Verification items for the finished model (mm, model axes). Give positions to 0.01 mm unless a question says otherwise; leave off trailing zeros. Write each loop counter-clockwise with the first axis right and the second up, starting at its lowest first coordinate (ties: lowest second). Pieces come first, ordered by that corner, then holes. Notation, with made-up numbers: (85.25, 78) - (119.25, 78) arc R36 ccw to (119.25, 116) - close; hole circle Ø10 at (-27, 52.25). An arc over 180 degrees is marked (long way). Put each result on its own line as item: value.
from build123d import *

# Parameters (mm, degrees)
F0_R     = 1
F0_R_2   = 0.8
F1_DEPTH = 1
F2_R     = 1


with BuildPart() as f1:
    # F0 (on Top) → F1 (new body)
    with BuildSketch(Plane.XY):
        Polygon((14.0690184001, 25), (0, 25), (-14.0690184001, 25), (-26.7296075576, 13.6899425008), (-24.0647631939, 10.7068896154), (-12.5425545984, 21), (0, 21), (12.5425545984, 21), (24.0647631939, 10.7068896154), (26.7296075576, 13.6899425008), align=None)
        with Locations((0, 23)):
            Circle(F0_R, mode=Mode.SUBTRACT)
        Polygon((28.9542586869, 11.7025995837), (26.7296075576, 13.6899425008), (24.0647631939, 10.7068896154), (26.2894143232, 8.7195466983), align=None)
        Polygon((-24.0647631939, 10.7068896154), (-26.7296075576, 13.6899425008), (-28.9542586869, 11.7025995837), (-26.2894143232, 8.7195466983), align=None)
        Polygon((31.3294992745, 9.5807309025), (28.9542586869, 11.7025995837), (26.2894143232, 8.7195466983), (27.3294992745, 7.7904097951), (27.3294992745, 0.0814010352), (27.3294992745, -0.0814010352), (27.3294992745, -7.7904097951), (26.2894143232, -8.7195466983), (28.9542586869, -11.7025995837), (31.3294992745, -9.5807309025), (31.3294992745, 0), align=None)
        with Locations((29.25, -7.3612159322)):
            Circle(F0_R_2, mode=Mode.SUBTRACT)
        with Locations((29.25, 7.3612159322)):
            Circle(F0_R_2, mode=Mode.SUBTRACT)
        Polygon((26.2894143232, 8.7195466983), (24.0647631939, 10.7068896154), (14.5, 0), (24.0647631939, -10.7068896154), (26.2894143232, -8.7195466983), (18.5, 0), align=None)
        with Locations((16.5, 0)):
            Circle(F0_R_2, mode=Mode.SUBTRACT)
        Polygon((-26.2894143232, 8.7195466983), (-28.9542586869, 11.7025995837), (-31.3294992745, 9.5807309025), (-31.3294992745, 0), (-31.3294992745, -9.5807309025), (-28.9542586869, -11.7025995837), (-26.2894143232, -8.7195466983), (-27.3294992745, -7.7904097951), (-27.3294992745, -0.0814010352), (-27.3294992745, 0.0814010352), (-27.3294992745, 7.7904097951), align=None)
        with Locations((-29.25, -7.3612159322)):
            Circle(F0_R_2, mode=Mode.SUBTRACT)
        with Locations((-29.25, 7.3612159322)):
            Circle(F0_R_2, mode=Mode.SUBTRACT)
        Polygon((-14.5, 0), (-24.0647631939, 10.7068896154), (-26.2894143232, 8.7195466983), (-18.5, 0), (-26.2894143232, -8.7195466983), (-24.0647631939, -10.7068896154), align=None)
        with Locations((-16.5, 0)):
            Circle(F0_R_2, mode=Mode.SUBTRACT)
        Polygon((26.2894143232, -8.7195466983), (24.0647631939, -10.7068896154), (26.7296075576, -13.6899425008), (28.9542586869, -11.7025995837), align=None)
        Polygon((26.7296075576, -13.6899425008), (24.0647631939, -10.7068896154), (12.5425545984, -21), (0, -21), (-12.5425545984, -21), (-24.0647631939, -10.7068896154), (-26.7296075576, -13.6899425008), (-14.0690184001, -25), (0, -25), (14.0690184001, -25), align=None)
        with Locations((0, -23)):
            Circle(F0_R, mode=Mode.SUBTRACT)
        Polygon((-26.7296075576, -13.6899425008), (-24.0647631939, -10.7068896154), (-26.2894143232, -8.7195466983), (-28.9542586869, -11.7025995837), align=None)
    extrude(amount=F1_DEPTH)

    # F2
    f2_edges = [f1.edges().sort_by_distance(p)[0] for p in [
        (-14.069018, 25, 0.5),
        (-31.329499, 9.580731, 0.5),
        (-31.329499, -9.580731, 0.5),
        (-14.069018, -25, 0.5),
        (14.069018, -25, 0.5),
        (31.329499, -9.580731, 0.5),
        (31.329499, 9.580731, 0.5),
        (14.069018, 25, 0.5),
        (14.5, 0, 0.5),
        (-14.5, 0, 0.5),
    ]]
    fillet(f2_edges, radius=F2_R)


solid = f1.part
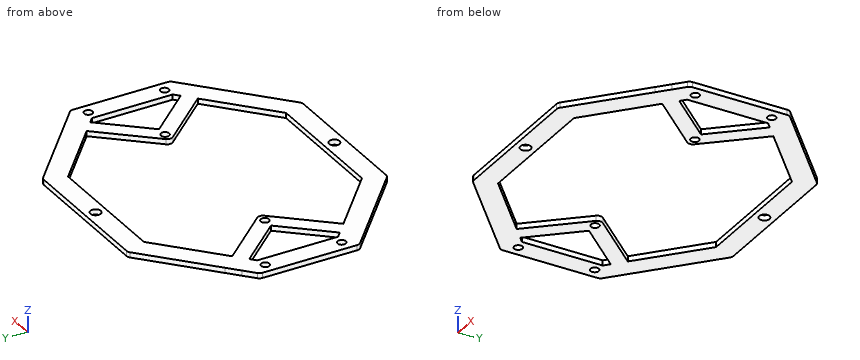
Q1. Section check D-D, the plane y = -4. Record the cut outline in (x, z), plus the area to 3 significant figures.
Answers follow:
outline: (-31.33, 0) - (-27.33, 0) - (-27.33, 1) - (-31.33, 1) - close; (-22.07, 0) - (-18.07, 0) - (-18.07, 1) - (-22.07, 1) - close; (18.07, 0) - (22.07, 0) - (22.07, 1) - (18.07, 1) - close; (27.33, 0) - (31.33, 0) - (31.33, 1) - (27.33, 1) - close
area: 16.0 mm2
Q2. Go/stop test with a flat-tipped pin: pin 1 Ø1 at (x, y) = (16.5, 0) entering from +Z. Record where the tip stops, or that it passes through.
Answers follow:
pin 1: passes through
Q3. Scan lines: line 1 along Y through (x, z) = (0, 0.25); line 2 along X through (y, z) = (-4, 0.55); line 3 along Y through (x, z) = (-8, 0.25). Record each from-to range of solid material in increasing order.
Answers follow:
line 1: y = -25 to -24, -22 to -21, 21 to 22, 24 to 25
line 2: x = -31.33 to -27.33, -22.07 to -18.07, 18.07 to 22.07, 27.33 to 31.33
line 3: y = -25 to -21, 21 to 25
Q4. Section check B-B, the plane x = -11. Record the cut outline in (y, z).
Answers follow:
outline: (-25, 0) - (-21, 0) - (-21, 1) - (-25, 1) - close; (21, 0) - (25, 0) - (25, 1) - (21, 1) - close
Q5. Section check C-C, the plane y = 23. Record the cut outline in (x, z), plus the area to 3 significant figures.
Answers follow:
outline: (-16.31, 0) - (-1, 0) - (-1, 1) - (-16.31, 1) - close; (1, 0) - (16.31, 0) - (16.31, 1) - (1, 1) - close
area: 30.6 mm2
Q6. Section check A-A, the plane x = 0. Record the cut outline in (y, z).
Answers follow:
outline: (-25, 0) - (-24, 0) - (-24, 1) - (-25, 1) - close; (-22, 0) - (-21, 0) - (-21, 1) - (-22, 1) - close; (21, 0) - (22, 0) - (22, 1) - (21, 1) - close; (24, 0) - (25, 0) - (25, 1) - (24, 1) - close
